```python
from build123d import *

# Parameters (mm, degrees)
SKETCH_1_R           = 29.5
SKETCH_1_R_2         = 2.25
EXTRUDE_1_DEPTH      = 2.5
EXTRUDE_2_DEPTH      = 2.5
SKETCH_3_W           = 2.5
SKETCH_3_H           = 20.5
SKETCH_3_H_2         = 29.5
EXTRUDE_3_DEPTH      = 42
SKETCH_4_W           = 15.5
SKETCH_4_H           = 42
SKETCH_4_W_2         = 6
CUT_EXTRUDE_1_DEPTH  = 60
SKETCH_5_R           = 4.3
EXTRUDE_4_DEPTH      = 2.5
CUT_EXTRUDE_9_DEPTH  = 122.813381989
EXTRUDE_6_DEPTH      = 2.5
SKETCH_14_R          = 4.3
CUT_EXTRUDE_10_DEPTH = 118.573381341
FILLET_3_R           = 9


with BuildPart() as part:
    # Sketch 1 → Extrude 1 (new body)
    with BuildSketch(Plane.XY):
        Polygon((0, 31.5), (31.5, 31.5), (31.5, -34), (-31.5, -34), (-31.5, 31.5), align=None)
        Circle(SKETCH_1_R, mode=Mode.SUBTRACT)
        with Locations((-26.516504294, 26.516504294)):
            Circle(SKETCH_1_R_2, mode=Mode.SUBTRACT)
        with Locations((26.516504294, 26.516504294)):
            Circle(SKETCH_1_R_2, mode=Mode.SUBTRACT)
        with Locations((26.516504294, -26.516504294)):
            Circle(SKETCH_1_R_2, mode=Mode.SUBTRACT)
        with Locations((-26.516504294, -26.516504294)):
            Circle(SKETCH_1_R_2, mode=Mode.SUBTRACT)
    extrude(amount=EXTRUDE_1_DEPTH)

    # Sketch 2 → Extrude 2 (add)
    with BuildSketch(Plane(origin=(0, -34, 0), x_dir=(1, 0, 0), z_dir=(0, 1, 0))):
        Polygon((-31.5, 46.5), (-31.5, -2.5), (-20, -2.5), (-20, -22.5), (20, -22.5), (20, -2.5), (31.5, -2.5), (31.5, 46.5), (20, 46.5), (20, 66.5), (-20, 66.5), (-20, 46.5), align=None)
    extrude(amount=EXTRUDE_2_DEPTH)

    # Sketch 3 → Extrude 3 (add)
    with BuildSketch(Plane(origin=(0, -31.5, 0), x_dir=(1, 0, 0), z_dir=(0, 1, 0))):
        with Locations((21.25, 56.25)):
            Rectangle(SKETCH_3_W, SKETCH_3_H)
        with Locations((-21.25, 56.25)):
            Rectangle(SKETCH_3_W, SKETCH_3_H)
        with Locations((-21.25, -7.75)):
            Rectangle(SKETCH_3_W, SKETCH_3_H_2)
        with Locations((21.25, -7.75)):
            Rectangle(SKETCH_3_W, SKETCH_3_H_2)
    extrude(amount=-EXTRUDE_3_DEPTH)

    # Sketch 4 → Cut-Extrude 1 (cut)
    with BuildSketch(Plane.ZY.offset(22.5)):
        with Locations((14.75, -52.5)):
            Rectangle(SKETCH_4_W, SKETCH_4_H)
        with Locations((-63.5, -52.5)):
            Rectangle(SKETCH_4_W_2, SKETCH_4_H)
    extrude(amount=-CUT_EXTRUDE_1_DEPTH, mode=Mode.SUBTRACT)

    # Sketch 5 → Extrude 4 (add)
    # profile 1 of 2: a face of its own
    with BuildSketch(Plane(origin=(0, -31.5, 0), x_dir=(1, 0, 0), z_dir=(0, 1, 0))):
        with BuildLine():
            Line((-31.5, 33.999994356), (-39.5, 33.999994356))
            ThreePointArc((-39.5, 33.999994356), (-46.499999777, 27.00176014), (-39.503531569, 19.999995247))
            Line((-39.503531569, 19.999995247), (-31.5, 19.999995247))
            Line((-31.5, 19.999995247), (-31.5, 33.999994356))
        make_face()
        with Locations(Location((-39.5, 26.999994356, 0), (0, 0, 270))):
            Circle(SKETCH_5_R, mode=Mode.SUBTRACT)
    # profile 2 of 2: a face of its own
    with BuildSketch(Plane(origin=(0, -31.5, 0), x_dir=(1, 0, 0), z_dir=(0, 1, 0))):
        with BuildLine():
            Line((44.500000207, 35.999994356), (31.5, 35.999994356))
            Line((31.5, 35.999994356), (31.5, 26.5))
            Line((31.5, 26.5), (31.5, 17.999994356))
            Line((31.5, 17.999994356), (44.500000207, 17.999994356))
            ThreePointArc((44.500000207, 17.999994356), (53.500000207, 26.999994356), (44.500000207, 35.999994356))
        make_face()
        with Locations(Location((46.5, 26.999994356, 0), (0, 0, 270))):
            Circle(SKETCH_5_R, mode=Mode.SUBTRACT)
    extrude(amount=-EXTRUDE_4_DEPTH)

    # Sketch 12 → Cut-Extrude 9 (cut, through all)
    with BuildSketch(Plane.ZY.offset(22.5)):
        Polygon((-46, -73.5), (-47, -73.5), (-47, -31.5), (-46.5, -31.5), (-46, -31.5), align=None)
    extrude(amount=-CUT_EXTRUDE_9_DEPTH, mode=Mode.SUBTRACT)


with BuildPart() as cut_extrude_9_piece_1:
    # of the separate pieces the step leaves, piece 1, a body of its own (cut_extrude_9_pieces)
    add(part.part.solids().sort_by_distance((31.5, 31.5, 0))[0])



with BuildPart() as cut_extrude_9_piece_2:
    # of the separate pieces the step leaves, piece 2, a body of its own (cut_extrude_9_pieces)
    add(part.part.solids().sort_by_distance((-22.5, -31.5, -60.5))[0])


with BuildPart() as cut_extrude_9_piece_1_1:
    add(cut_extrude_9_piece_1.part)

    add(cut_extrude_9_piece_2.part)  # Extrude 6 merges Cut-Extrude 9 piece 2
    # Sketch 13 → Extrude 6 (add)
    with BuildSketch(Plane(origin=(0, -31.5, 0), x_dir=(1, 0, 0), z_dir=(0, 1, 0))):
        Polygon((31.5, 46.5), (31.5, 47), (22.5, 47), (-22.5, 47), (-31.5, 47), (-31.5, 46.5), (-22.5, 46.5), (-22.5, 46), (31.5, 46), align=None)
    extrude(amount=-EXTRUDE_6_DEPTH)

    # Sketch 14 → Cut-Extrude 10 (cut, through all)
    with BuildSketch(Plane(origin=(22.5, 0, 0), x_dir=(0, 0, -1), z_dir=(1, 0, 0))):
        with Locations((0, -53.5)):
            Circle(SKETCH_14_R)
        with Locations((53.75, -53.5)):
            Circle(SKETCH_14_R)
    extrude(amount=-CUT_EXTRUDE_10_DEPTH, mode=Mode.SUBTRACT)

    # Fillet 3
    fillet_3_edges = [cut_extrude_9_piece_1_1.edges().sort_by_distance(p)[0] for p in [
        (-31.5, -32.75, -47),
        (31.5, -32.75, -47),
    ]]
    fillet(fillet_3_edges, radius=FILLET_3_R - 0.0001)  # a hair under: the kernel refuses the full size


solid = cut_extrude_9_piece_1_1.part
```
The model under review builds one solid part; all positions refer to its coordinate system, in mm. A direction names the side the tool comes from. Give positions to 0.01 mm unless a question says otherwise; leave off trailing zeros. Write each loop counter-clockwise with the first axis right and the second up, starting at its lowest first coordinate (ties: lowest second). Pieces come first, ordered by that corner, then holes. Notation, with made-up numbers: M -20.75,63 L -16.75,63 A21 ccw -16.75,68 Z; hole C 13,53 d6. An arc over 180 degrees is marked long. Answer in a Markdown table with one row per item.
Item 1: For line 1 along X through (y, z) = (-45, -1.5); line 2 along Y through (x, z) = (15, -40); line 3 along Y through (x, z) = (22, -5), list the stretches that pass through material, from the lowest coordinate up.
Check sheet entries:
| item | result |
|---|---|
| line 1 | -22.5 to -20, 20 to 22.5 |
| line 2 | -34 to -31.5 |
| line 3 | -73.5 to -31.5 |
Item 2: Add section C-C on x = 0. Give the boundary of the cut face in (y, z), plus the area to 3 significant figures.
Check sheet entries:
| item | result |
|---|---|
| outline | M -34,-60.5 L -31.5,-60.5 L -31.5,0 L -29.5,0 L -29.5,2.5 L -31.5,2.5 L -31.5,7 L -34,7 Z; M 29.5,0 L 31.5,0 L 31.5,2.5 L 29.5,2.5 Z |
| area | 179 mm2 |
Item 3: Add section A-A on z = -53.75. Give the boundary of the cut face in (x, y), plus the area to 3 significant figures.
Check sheet entries:
| item | result |
|---|---|
| outline | M -22.5,-73.5 L -20,-73.5 L -20,-57.8 L -22.5,-57.8 Z; M -22.5,-49.2 L -20,-49.2 L -20,-34 L 20,-34 L 20,-49.2 L 22.5,-49.2 L 22.5,-31.5 L -22.5,-31.5 Z; M 20,-73.5 L 22.5,-73.5 L 22.5,-57.8 L 20,-57.8 Z |
| area | 267 mm2 |
Item 4: Add section B-B on y = 0. Give the boundary of the cut face in (x, z).
Check sheet entries:
| item | result |
|---|---|
| outline | M -31.5,0 L -29.5,0 L -29.5,2.5 L -31.5,2.5 Z; M 29.5,0 L 31.5,0 L 31.5,2.5 L 29.5,2.5 Z |
Item 5: Draft analysis for pull direction Z (two halves, no side actions). For faces 4 (the face through (-36, -33, -20)), 5 (the face through (-20, -58, -54)), 6 (the face through (-46.5, -32.73, -27.16)), 7 (the face through (-21, -53, -7)), state which applies: +Z half, -Z half, draft (parallel to the pull), parting line (faces both ways), or undercut.
Check sheet entries:
| item | result |
|---|---|
| face 4 | +Z half |
| face 5 | draft |
| face 6 | parting line |
| face 7 | undercut |
Item 6: Add section D-D on y = -66. Give the boundary of the cut face in (x, z).
Check sheet entries:
| item | result |
|---|---|
| outline | M -22.5,-60.5 L -20,-60.5 L -20,-47 L -22.5,-47 Z; M -22.5,-7 L -20,-7 L -20,7 L -22.5,7 Z; M 20,-60.5 L 22.5,-60.5 L 22.5,-47 L 20,-47 Z; M 20,-7 L 22.5,-7 L 22.5,7 L 20,7 Z |
Item 7: For P1, Ø2, axis at x = 36.5, y = -32.5, coming from the +Z side; P2, Ø1.2, axis at y = -33, z = -36.5, coming from the -X side; P3, Ø2, axis at x = 3.5, z = -27.5, coming from the -Y side, all flat-tipped, find the tip position at first contact; note any pin that passes through.
Check sheet entries:
| item | result |
|---|---|
| P1 | z = -18 |
| P2 | x = -31.5 |
| P3 | y = -34 |
Item 8: Tool access review of faces 1 (the face through (38, -33, -18)), 2 (the face through (-22.5, -48, -54)), 3 (the face through (38, -33, -36)): name each direction out of +Z, -Z, +X, -X, +Y, -Y from which nothing blocks a thin tool from reaching the whole face with its end or side.
Check sheet entries:
| item | result |
|---|---|
| face 1 | +Z, +X, +Y, -Y |
| face 2 | -Z, -X, +Y, -Y |
| face 3 | -Z, +X, +Y, -Y |
